Geometry: final body of the model. Coordinates: model frame, mm. Face numbers are marked on the shaded views. A direction names the side the tool comes from. Coordinates: 2 decimals unless noted, no trailing zeros. Loops run counter-clockwise (first coordinate to the right, second up) from the corner with the lowest first, then second, coordinate; pieces in that order, holes last. Notation, with made-up numbers: (38, 56) -> (43, 56) arc R23 cw to (43, 87) -> close; hole circle Ø7 at (-8, -13.75). An arc over 180 degrees is marked (long way). One line per item, written item: value. Start each with the question number.
Item 1: Section query A-A on y = -13.5. Return loops of the section in (x, z), then the cut area to 3 significant figures.
Item 2: Section query B-B on x = -54. Return loops of the section in (y, z), then the cut area to 3 significant figures.
Item 3: Ray query, probe 1 along X at (y, z) = (-15.5, 24.5); probe 2 along X at (y, z) = (-23, 29); probe 3 along Z at (x, y) = (-41.5, -4). Return the intervals inside material, ascending. Write a range as from..to.
Item 4: Set-up query: the marked faces 1 and 2. Return all of +Z, -Z, +X, -X, +Y, -Y with unobstructed straight access to the full face (end or side cutting, diameter ignored); none if empty.
Item 5: Section query C-C on z = 51. Return loops of the section in (x, y), then the cut area to 3 significant figures.
Item 6: Section query D-D on z = 42. Return loops of the section in (x, y), then the cut area to 3 significant figures.
Item 7: Contact query for flat-ended pins moving along their axis: pin 1 Ø10 at (y, z) = (-25, -10.5) entering from +X; pin 2 Ø12 at (y, z) = (-27.5, 23.5) entering from +X. Output: stop coordinate, or through.
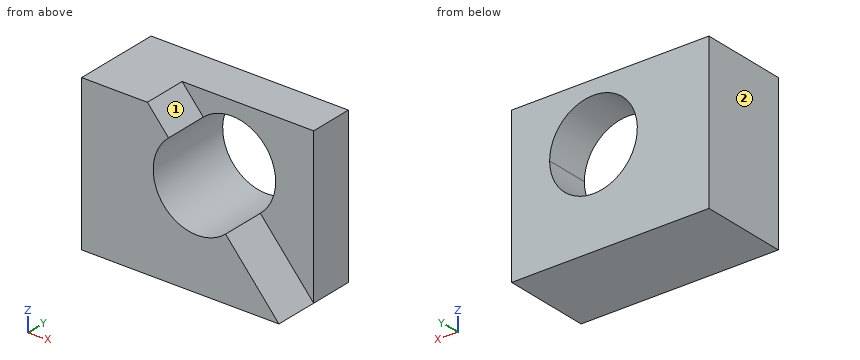
from build123d import *

# Parameters (mm, degrees)
F0_W     = 25.4
F0_H     = 88.9
F1_DEPTH = 114.3
F3_DEPTH = 25.4
F5_DEPTH = 50.801


with BuildPart() as f1:
    # F0 (on Right) → F1 (new body)
    with BuildSketch(Plane.YZ):
        with Locations((-2.9790955596, 18.0637241125)):
            Rectangle(F0_W, F0_H)
    extrude(amount=-F1_DEPTH)

    # F2 (on face) → F3 (join)
    with BuildSketch(Plane.XZ.offset(15.6790955596)):
        Polygon((-76.2, 62.5137241125), (-114.3, 62.5137241125), (-114.3, -26.3862758875), (0, -26.3862758875), align=None)
    extrude(amount=F3_DEPTH)

    # F4 (on face) → F5 (cut, through all)
    with BuildSketch(Plane.XZ.offset(41.0790955596)):
        with BuildLine():
            Line((-30.8922379172, 9.6546683493), (-63.9524396888, 48.2249037495))
            ThreePointArc((-63.9524396888, 48.2249037495), (-66.7074565031, 12.4096851636), (-30.8922379172, 9.6546683493))
        make_face()
        with BuildLine():
            ThreePointArc((-30.8922379172, 9.6546683493), (-24.3461111813, 18.3262230873), (-22.022338803, 28.9397860494))
            ThreePointArc((-22.022338803, 28.9397860494), (-36.8087758409, 52.0160136711), (-63.9524396888, 48.2249037495))
            Line((-63.9524396888, 48.2249037495), (-30.8922379172, 9.6546683493))
        make_face()
    extrude(amount=-F5_DEPTH, mode=Mode.SUBTRACT)


solid = f1.part
Reply:
1. outline: (-114.3, -26.39) -> (0, -26.39) -> (0, 62.51) -> (-114.3, 62.51) -> close; hole circle Ø50.8 at (-47.42, 28.94)
1. area: 8,130 mm²
2. outline: (-41.08, -26.39) -> (9.72, -26.39) -> (9.72, 4.41) -> (-41.08, 4.41) -> close; (-15.68, 53.47) -> (9.72, 53.47) -> (9.72, 62.51) -> (-15.68, 62.51) -> close
2. area: 1,790 mm²
3. probe 1: x = -114.3..-72.43, -22.41..0
3. probe 2: x = -114.3..-72.82
3. probe 3: z = -26.39..4.24, 53.64..62.51
4. face 1: +Z, +X, -Y
4. face 2: +Z, -Z, -X, +Y, -Y
5. outline: (-114.3, -41.08) -> (-66.33, -41.08) -> (-66.33, -15.68) -> (-60.01, -15.68) -> (-60.01, 9.72) -> (-114.3, 9.72) -> close; (-34.83, -15.68) -> (0, -15.68) -> (0, 9.72) -> (-34.83, 9.72) -> close
5. area: 3,480 mm²
6. outline: (-114.3, -41.08) -> (-69.21, -41.08) -> (-69.21, 9.72) -> (-114.3, 9.72) -> close; (-25.64, -15.68) -> (0, -15.68) -> (0, 9.72) -> (-25.64, 9.72) -> close
6. area: 2,940 mm²
7. pin 1: stops at x = -9.33
7. pin 2: stops at x = -70.1
